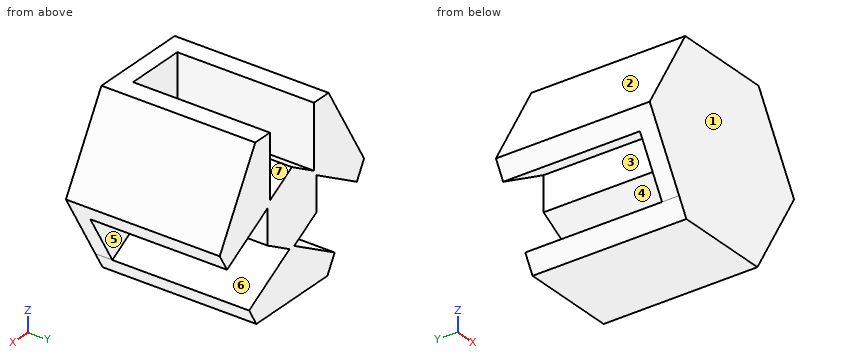
```python
from build123d import *

# Parameters (mm, degrees)
F2_DEPTH = 3.175
F3_DEPTH = 25.4


# Not quite as in the source:
# - a feature names something its author has since deleted; it is built from what else it names


with BuildPart() as f2:
    # F1 (on Front) → F2 (new body)
    with BuildSketch(Plane.XZ):
        Polygon((-18.1618179038, 0.1631008549), (-16.3287307991, -3.0118991451), (-6.1622247723, 2.8577358462), (-6.1622247723, 3.5577621311), (-5.5559842263, 3.9077752735), (-5.5559842263, 15.6470452561), (-9.2221584356, 15.6470452561), align=None)
        Polygon((6.1622247723, 2.8577358462), (16.3287307991, -3.0118991451), (18.1618179038, 0.1631008549), (9.2221584356, 15.6470452561), (5.5559842263, 15.6470452561), (5.5559842263, 3.9077752735), (6.1622247723, 3.5577621311), align=None)
        Polygon((-0.606240546, -6.7655111197), (-10.7727465728, -12.635146111), (-8.9396594682, -15.810146111), (8.9396594682, -15.810146111), (10.7727465728, -12.635146111), (0.606240546, -6.7655111197), (0, -7.1155242622), align=None)
        Polygon((5.5559842263, 3.2077489886), (6.1622247723, 2.8577358462), (6.1622247723, 3.5577621311), (5.5559842263, 3.9077752735), align=None)
        Polygon((-6.1622247723, 3.5577621311), (-6.1622247723, 2.8577358462), (-5.5559842263, 3.2077489886), (-5.5559842263, 3.9077752735), align=None)
        Polygon((0, -6.4154979773), (-0.606240546, -6.7655111197), (0, -7.1155242622), (0.606240546, -6.7655111197), align=None)
        Polygon((-6.1622247723, -3.5577621311), (-0.606240546, -6.7655111197), (0, -6.4154979773), (0.606240546, -6.7655111197), (6.1622247723, -3.5577621311), (6.1622247723, 2.8577358462), (5.5559842263, 3.2077489886), (5.5559842263, 3.9077752735), (0, 7.1155242622), (-5.5559842263, 3.9077752735), (-5.5559842263, 3.2077489886), (-6.1622247723, 2.8577358462), align=None)
        Polygon((5.5559842263, 15.6470452561), (-5.5559842263, 15.6470452561), (-5.5559842263, 3.9077752735), (0, 7.1155242622), (5.5559842263, 3.9077752735), align=None)
        Polygon((-16.3287307991, -3.0118991451), (-10.7727465728, -12.635146111), (-0.606240546, -6.7655111197), (-6.1622247723, -3.5577621311), (-6.1622247723, 2.8577358462), align=None)
        Polygon((0.606240546, -6.7655111197), (10.7727465728, -12.635146111), (16.3287307991, -3.0118991451), (6.1622247723, 2.8577358462), (6.1622247723, -3.5577621311), align=None)
    extrude(amount=F2_DEPTH)

    # F1 (on Front) → F3 (join)
    with BuildSketch(Plane.XZ):
        Polygon((-18.1618179038, 0.1631008549), (-16.3287307991, -3.0118991451), (-6.1622247723, 2.8577358462), (-6.1622247723, 3.5577621311), (-5.5559842263, 3.9077752735), (-5.5559842263, 15.6470452561), (-9.2221584356, 15.6470452561), align=None)
        Polygon((-0.606240546, -6.7655111197), (-10.7727465728, -12.635146111), (-8.9396594682, -15.810146111), (8.9396594682, -15.810146111), (10.7727465728, -12.635146111), (0.606240546, -6.7655111197), (0, -7.1155242622), align=None)
        Polygon((6.1622247723, 2.8577358462), (16.3287307991, -3.0118991451), (18.1618179038, 0.1631008549), (9.2221584356, 15.6470452561), (5.5559842263, 15.6470452561), (5.5559842263, 3.9077752735), (6.1622247723, 3.5577621311), align=None)
        Polygon((-6.1622247723, -3.5577621311), (-0.606240546, -6.7655111197), (0, -6.4154979773), (0.606240546, -6.7655111197), (6.1622247723, -3.5577621311), (6.1622247723, 2.8577358462), (5.5559842263, 3.2077489886), (5.5559842263, 3.9077752735), (0, 7.1155242622), (-5.5559842263, 3.9077752735), (-5.5559842263, 3.2077489886), (-6.1622247723, 2.8577358462), align=None)
        Polygon((5.5559842263, 3.2077489886), (6.1622247723, 2.8577358462), (6.1622247723, 3.5577621311), (5.5559842263, 3.9077752735), align=None)
        Polygon((0, -6.4154979773), (-0.606240546, -6.7655111197), (0, -7.1155242622), (0.606240546, -6.7655111197), align=None)
        Polygon((-6.1622247723, 3.5577621311), (-6.1622247723, 2.8577358462), (-5.5559842263, 3.2077489886), (-5.5559842263, 3.9077752735), align=None)
    extrude(amount=-F3_DEPTH)


solid = f2.part
```
CAD build for the part. Positions are in the model's coordinates, mm. Face numbers are marked on the shaded views. A direction names the side the tool comes from. Round coordinates to 2 decimals unless told otherwise and drop trailing zeros. Loops run counter-clockwise (first coordinate to the right, second up) from the corner with the lowest first, then second, coordinate; pieces in that order, holes last. Notation, with made-up numbers: (17.5, 74) - (70.5, 74) arc R16 ccw to (70.5, 94) - close; hole circle Ø10 at (66.25, -5). An arc over 180 degrees is marked (long way). Return JSON: item names as keys, results as strings. Group by question number.
Q1. Band-saw the part on B-B on y = 9.5. Give the cut face in (x, z), plus the area to 3 significant figures.
Q2. Two-plate mould, pull along Z, no slides. Class the marked faces 1, 2 and 3: +Z half, -Z half, draft (parallel to the pull), parting line (faces both ways), or undercut.
Q3. Tool access for the marked faces 4, 5, 6 and 7: list every direction of +Z, -Z, +X, -X, +Y, -Y with a clear straight run to the whole face (end or side of a thin tool).
Q4. Drill centre lines: line 1 along X through (y, z) = (7.25, -1.5); line 2 along Y through (x, z) = (-12.5, -2) (3 decimals); line 3 along X through (y, z) = (2.75, -0.5). Where is each one in solid material? Low to high. Write a range as [from, to].
Q5. Band-saw the part on D-D on x = -14.5. Give the cut face in (y, z) (3 decimals).
Q6. Band-saw the part on A-A on x = 10. Give the cut face in (y, z) (3 decimals).
Q7. Band-saw the part on C-C on z = 9. Give the cut face in (x, y) (3 decimals), plus the area to 3 significant figures.
Q8. Flat gauge pins, fed straight in: pin 1 Ø12 at (y, z) = (18, 7) entering from +X; pin 2 Ø6 at (y, z) = (15, 10.5) entering from -X; pin 3 Ø5 at (y, z) = (9, 0) entering from +X. Where does each tip first touch, or does it go through?
Solutions:
{
 "1": {"outline": "(-18.16, 0.16) - (-16.33, -3.01) - (-6.16, 2.86) - (-6.16, -3.56) - (-0.61, -6.77) - (-10.77, -12.64) - (-8.94, -15.81) - (8.94, -15.81) - (10.77, -12.64) - (0.61, -6.77) - (6.16, -3.56) - (6.16, 2.86) - (16.33, -3.01) - (18.16, 0.16) - (9.22, 15.65) - (5.56, 15.65) - (5.56, 3.91) - (0, 7.12) - (-5.56, 3.91) - (-5.56, 15.65) - (-9.22, 15.65) - close", "area": "519 mm^2"},
 "2": {"face 1": "draft", "face 2": "+Z half", "face 3": "undercut"},
 "3": {"face 4": "-X, +Y", "face 5": "+Y", "face 6": "+X, +Y", "face 7": "+Z, +Y"},
 "4": {"line 1": "x = [-17.2, -13.71], [-6.16, 6.16], [13.71, 17.2]", "line 2": "y = [-3.175, 0]", "line 3": "x = [-17.78, -11.98], [-6.16, 6.16], [11.98, 17.78]"},
 "5": {"outline": "(-3.175, -6.179) - (0, -6.179) - (0, -1.956) - (25.4, -1.956) - (25.4, 6.506) - (-3.175, 6.506) - close"},
 "6": {"outline": "(-3.175, -13.974) - (25.4, -13.974) - (25.4, -12.189) - (0, -12.189) - (0, 0.642) - (25.4, 0.642) - (25.4, 14.3) - (-3.175, 14.3) - close"},
 "7": {"outline": "(-13.06, -3.175) - (13.06, -3.175) - (13.06, 25.4) - (5.556, 25.4) - (5.556, 0) - (-5.556, 0) - (-5.556, 25.4) - (-13.06, 25.4) - close", "area": "464 mm^2"},
 "8": {"pin 1": "stops at x = 17.68", "pin 2": "stops at x = -13.93", "pin 3": "stops at x = 18.16"}
}
